Geometry check sheet. Reference: the model listing, model coordinates, mm. Give positions to 0.01 mm unless a question says otherwise; leave off trailing zeros. Write each loop counter-clockwise with the first axis right and the second up, starting at its lowest first coordinate (ties: lowest second). Pieces come first, ordered by that corner, then holes. Notation, with made-up numbers: (52.5, -14) -> (64.5, -14) arc R7 cw to (64.5, -3) -> close; hole circle Ø11 at (3.25, 56). An arc over 180 degrees is marked (long way). One line per item, written item: value.
from build123d import *

# Parameters (mm, degrees)
ESBO_O2_W                = 53
ESBO_O2_H                = 100
RESSALTO_EXTRUS_O1_DEPTH = 3
ESBO_O14_R               = 2
CORTE_EXTRUS_O10_DEPTH   = 10
ESBO_O8_R                = 5
CORTE_EXTRUS_O11_DEPTH   = 10
ESBO_O4_R                = 2
CORTE_EXTRUS_O12_DEPTH   = 10


with BuildPart() as part:
    # Esboço2 → Ressalto-extrusão1 (new body)
    with BuildSketch(Plane(origin=(-2.802903092, 0, -5.758743908), x_dir=(1, 0, 0), z_dir=(0, 1, 0))):
        with Locations((-26.430669922, 50)):
            Rectangle(ESBO_O2_W, ESBO_O2_H)
    extrude(amount=RESSALTO_EXTRUS_O1_DEPTH)

    # Esboço14 → Corte-extrusão10 (cut)
    with BuildSketch(Plane(origin=(0, 3, 0), x_dir=(1, 0, 0), z_dir=(0, 1, 0))):
        with Locations(Location((-27.802903092, 15.758743908, 0), (0, 0, 270))):
            Circle(ESBO_O14_R)
    extrude(amount=-CORTE_EXTRUS_O10_DEPTH, mode=Mode.SUBTRACT)

    # Esboço8 → Corte-extrusão11 (cut)
    with BuildSketch(Plane(origin=(0, 3, 0), x_dir=(1, 0, 0), z_dir=(0, 1, 0))):
        with Locations(Location((-40, 25, 0), (0, 0, 270))):
            Circle(ESBO_O8_R)
        with Locations(Location((-40, 36, 0), (0, 0, 270))):
            Circle(ESBO_O8_R)
        with Locations(Location((-40, 47.07, 0), (0, 0, 270))):
            Circle(ESBO_O8_R)
        with Locations(Location((-40, 58.07, 0), (0, 0, 270))):
            Circle(ESBO_O8_R)
        with Locations(Location((-40, 69, 0), (0, 0, 270))):
            Circle(ESBO_O8_R)
        with Locations(Location((-40, 80, 0), (0, 0, 270))):
            Circle(ESBO_O8_R)
    extrude(amount=-CORTE_EXTRUS_O11_DEPTH, mode=Mode.SUBTRACT)

    # Esboço4 → Corte-extrusão12 (cut)
    with BuildSketch(Plane(origin=(0, 3, 0), x_dir=(1, 0, 0), z_dir=(0, 1, 0))):
        with Locations(Location((-27.802903092, 96, 0), (0, 0, 270))):
            Circle(ESBO_O4_R)
    extrude(amount=-CORTE_EXTRUS_O12_DEPTH, mode=Mode.SUBTRACT)


solid = part.part
1) Mould release check, pull along Z, two halves, no side actions. Record for faces 1 (the cylindrical face through (-37, 2, -29)), 2 (the cylindrical face through (-29.02, 1.521, -17.346)), 3 (the flat face through (-30, 1, -5.759)), 4 (the flat face through (-55.734, 1, -55)): released by +Z, released by -Z, zero draft, split by the parting line, or undercut.
Verdict:
face 1: undercut
face 2: undercut
face 3: released by +Z
face 4: zero draft
2) Sectioned sample at B-B on x = -40. Record the cut outline in (y, z), plus the area to 3 significant figures.
Verdict:
outline: (0, -105.76) -> (3, -105.76) -> (3, -85) -> (0, -85) -> close; (0, -75) -> (3, -75) -> (3, -74) -> (0, -74) -> close; (0, -64) -> (3, -64) -> (3, -63.07) -> (0, -63.07) -> close; (0, -53.07) -> (3, -53.07) -> (3, -52.07) -> (0, -52.07) -> close; (0, -42.07) -> (3, -42.07) -> (3, -41) -> (0, -41) -> close; (0, -31) -> (3, -31) -> (3, -30) -> (0, -30) -> close; (0, -20) -> (3, -20) -> (3, -5.76) -> (0, -5.76) -> close
area: 120 mm^2
3) Sectioned sample at C-C on y = 2.5. Give the number of separate pieces and of enclosed holes in the cut face, plus the area to 3 significant figures.
Verdict:
separate pieces: 1
enclosed holes: 8
area: 4,800 mm^2
4) Depth check by flat-ended pin: pin 1 Ø9 at (x, z) = (-40, -69) entering from -Y. Enter the tip coordinate at first touch or a pass-through.
Verdict:
pin 1: through
5) Scan lines: probe 1 along X at (y, z) = (2.1, -36); probe 2 along X at (y, z) = (0.4, -35). Record each from-to range of solid material in increasing order.
Verdict:
probe 1: -55.73 to -45, -35 to -2.73
probe 2: -55.73 to -44.9, -35.1 to -2.73
6) Sectioned sample at A-A on z = -84. Record the cut outline in (x, y), plus the area to 3 significant figures.
Verdict:
outline: (-55.73, 0) -> (-43, 0) -> (-43, 3) -> (-55.73, 3) -> close; (-37, 0) -> (-2.73, 0) -> (-2.73, 3) -> (-37, 3) -> close
area: 141 mm^2
7) Sectioned sample at D-D on z = -58.07. Record the cut outline in (x, y).
Verdict:
outline: (-55.73, 0) -> (-45, 0) -> (-45, 3) -> (-55.73, 3) -> close; (-35, 0) -> (-2.73, 0) -> (-2.73, 3) -> (-35, 3) -> close
